Job drawing, mm, ordinate dimensions from the low corner. One solid piece. Round coordinates to 2 decimals unless told otherwise and drop trailing zeros. Write each loop counter-clockwise with the first axis right and the second up, starting at its lowest first coordinate (ties: lowest second). Pieces come first, ordered by that corner, then holes. Notation, with made-up numbers: M 62,-28.75 L 94,-28.75 A25 cw 94,-10.75 Z; hole C 42.25,0 d3. An arc over 180 degrees is marked long. Write each question's results on one line, items separated by ' | '. Start each with the question number.
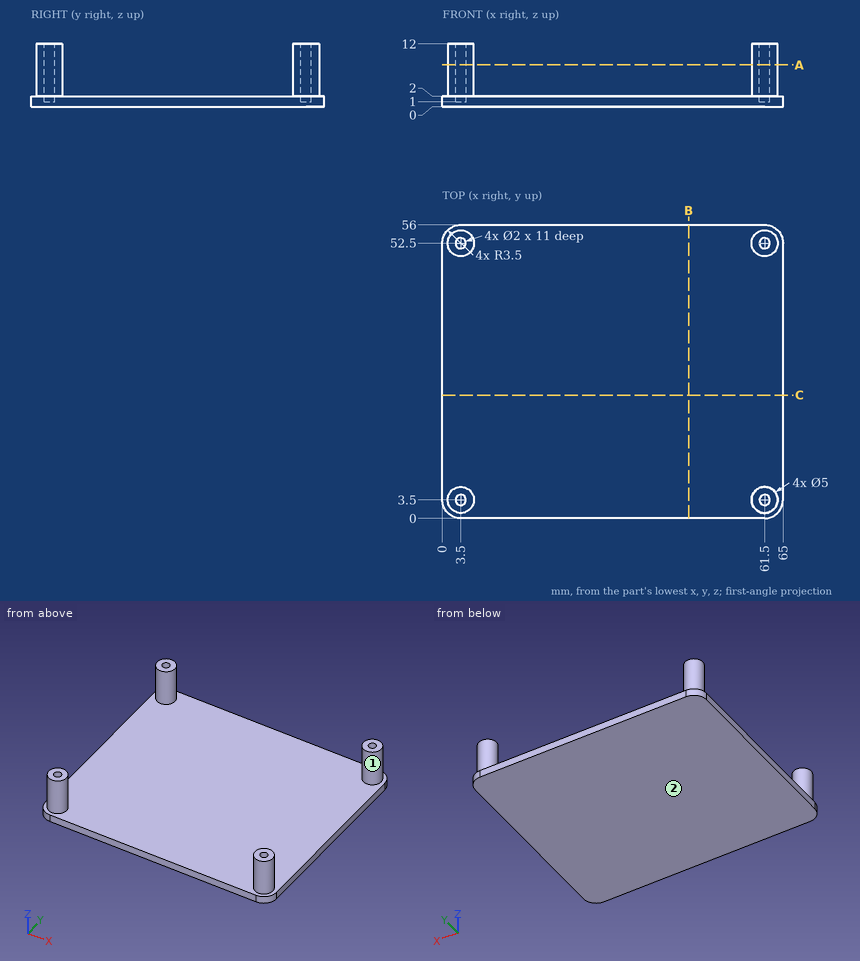
1) Saw through at C-C, the plane y = 23.5. Write the cut outline in (x, z), plus the area to 3 significant figures.
2) Saw through at B-B, the plane x = 47. Write the cut outline in (y, z).
3) Pull direction Y, two halves, no side cores. Call the marked faces 1 and 2: pulls with the +Y half, pulls with the -Y half, needs draft (parallel to the pull), parting line crosses it, or undercut.
4) Drop flat-ended pins along their axis: pin 1 Ø1.6 at (x, y) = (61.5, 3.5) entering from +Z; pin 2 Ø10 at (x, y) = (42.5, 34.5) entering from +Z. Give the stop position or say it passes through.
5) Saw through at A-A, the plane z = 8. Write the cut outline in (x, y), plus the area to 3 significant figures.
6) Wall check: line 1 along X through (y, z) = (3.5, 8); line 2 along Y through (x, z) = (3.5, 7.5); line 3 along Z through (x, y) = (31.5, 14.5). Give the ranges that are in metal, low to high. Write a range as from..to.
Filled sheet:
1) outline: M 0,0 L 65,0 L 65,2 L 0,2 Z | area: 130 mm^2
2) outline: M 0,0 L 56,0 L 56,2 L 0,2 Z
3) face 1: undercut | face 2: needs draft
4) pin 1: stops at z = 1 | pin 2: stops at z = 2
5) outline: C 3.5,3.5 d5; C 3.5,52.5 d5; C 61.5,3.5 d5; C 61.5,52.5 d5; hole C 3.5,3.5 d2; hole C 3.5,52.5 d2; hole C 61.5,3.5 d2; hole C 61.5,52.5 d2 | area: 66.0 mm^2
6) line 1: x = 1..2.5, 4.5..6, 59..60.5, 62.5..64 | line 2: y = 1..2.5, 4.5..6, 50..51.5, 53.5..55 | line 3: z = 0..2
